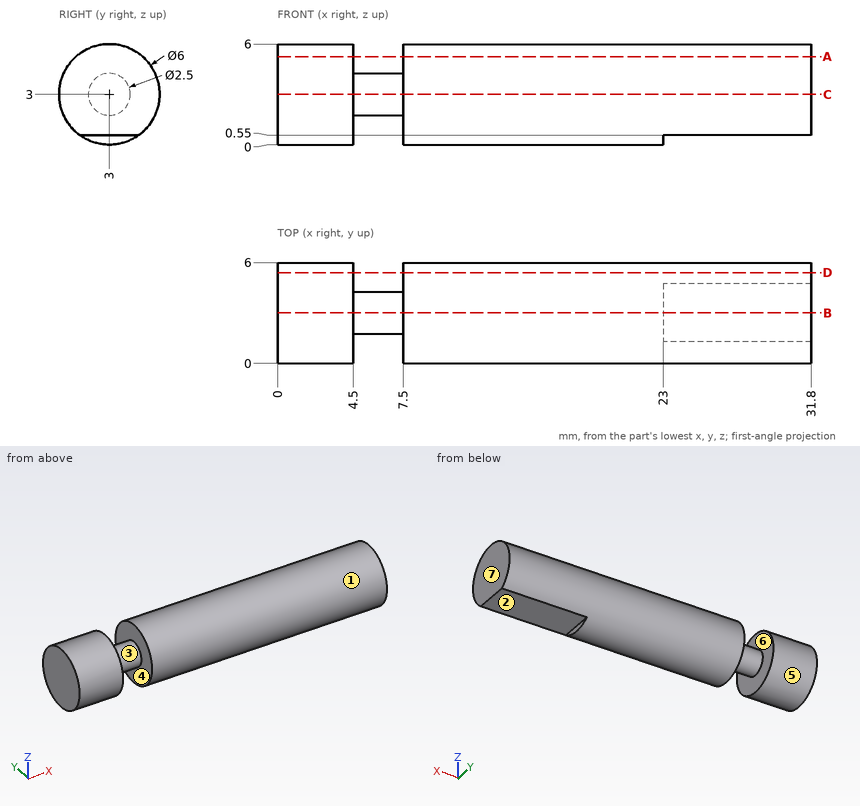
For this review, use the dimensioned drawing (mm, ordinates from the lowest corner) and the shaded views. A direction names the side the tool comes from. Round coordinates to 2 decimals unless told otherwise and drop trailing zeros. Order: outer loops, then holes, each group sorted by start corner. A loop starts at its lowest first (then second) coordinate and runs counter-clockwise, first axis right, second up. Notation, with made-up numbers: M 72.25,10 L 89.25,10 A23 ccw 89.25,37 Z; hole C 86.25,-27.75 d8. An arc over 180 degrees is marked long. Use a Markdown table: item, result. Add a question column.
Item 1: Add section B-B, the plane y = 3. Give the boundary of the cut face in (x, z), then the cut area to 3 significant figures.
Item 2: Add section C-C, the plane z = 3. Give the boundary of the cut face in (x, y), then the cut area to 3 significant figures.
Item 3: To check wall thickness, follow line 1 along X through (y, z) = (0.85, 2.65); line 2 along X through (y, z) = (3, 0.25); line 3 along Y through (x, z) = (14, 3.2). State the ranges of each line that lie inside material, in increasing order.
Item 4: Add section A-A, the plane z = 5.25. Give the boundary of the cut face in (x, y), then the cut area to 3 significant figures.
Item 5: Mouldability with a two-part tool opening along X and no side actions: class the marked faces 4, 5, 6 and 7 as released by +X, released by -X, zero draft, split by the parting line, or undercut.
Item 6: Add section D-D, the plane y = 5.4. Give the boundary of the cut face in (x, z), then the cut area to 3 significant figures.
Item 7: Tool access review of the marked faces 1, 2 and 3: name each direction out of +Z, -Z, +X, -X, +Y, -Y from which nothing blocks a thin tool from reaching the whole face with its end or side.
Item 8: Insertion check: pin 1 (1.8 mm diameter, centred on y = 2.5, z = 2.5, fed in from -X); pin 2 (1 mm diameter, centred on x = 26.5, y = 3.5, fed in from -Z). Each pin has a flat end and moves straight along its axis. Give the tip position at first contact, or say it passes through.
Geometry results:
| question | item | result |
|---|---|---|
| 1 | outline | M 0,0 L 4.5,0 L 4.5,1.75 L 7.5,1.75 L 7.5,0 L 23,0 L 23,0.55 L 31.8,0.55 L 31.8,6 L 7.5,6 L 7.5,4.25 L 4.5,4.25 L 4.5,6 L 0,6 Z |
| 1 | area | 175 mm² |
| 2 | outline | M 0,0 L 4.5,0 L 4.5,1.75 L 7.5,1.75 L 7.5,0 L 31.8,0 L 31.8,6 L 7.5,6 L 7.5,4.25 L 4.5,4.25 L 4.5,6 L 0,6 Z |
| 2 | area | 180 mm² |
| 3 | line 1 | x = 0 to 4.5, 7.5 to 31.8 |
| 3 | line 2 | x = 0 to 4.5, 7.5 to 23 |
| 3 | line 3 | y = 0.01 to 5.99 |
| 4 | outline | M 0,1.02 L 4.5,1.02 L 4.5,4.98 L 0,4.98 Z; M 7.5,1.02 L 31.8,1.02 L 31.8,4.98 L 7.5,4.98 Z |
| 4 | area | 114 mm² |
| 5 | face 4 | undercut |
| 5 | face 5 | zero draft |
| 5 | face 6 | undercut |
| 5 | face 7 | released by +X |
| 6 | outline | M 0,1.2 L 4.5,1.2 L 4.5,4.8 L 0,4.8 Z; M 7.5,1.2 L 31.8,1.2 L 31.8,4.8 L 7.5,4.8 Z |
| 6 | area | 104 mm² |
| 7 | face 1 | +X, -X |
| 7 | face 2 | -Z, +X, +Y, -Y |
| 7 | face 3 | none |
| 8 | pin 1 | stops at x = 0 |
| 8 | pin 2 | stops at z = 0.55 |
